from build123d import *

# Parameters (mm, degrees)
F1_DEPTH = 154
F3_D     = 2.7
F3_DEPTH = 12
F3_TIP   = 0.8111618357
F4_W     = 154
F4_H     = 12
F5_DEPTH = 1
F6_W     = 154
F6_H     = 12
F7_DEPTH = 1


with BuildPart() as f1:
    # F0 (on Front) → F1 (new body)
    with BuildSketch(Plane.XZ):
        with BuildLine():
            Line((-10.0352883258, -17.0069661875), (0, -17.0069661875))
            Line((0, -17.0069661875), (10.0352883258, -17.0069661875))
            Line((10.0352883258, -17.0069661875), (7, -12.5069661875))
            Line((7, -12.5069661875), (46.25, -12.5069661875))
            Line((46.25, -12.5069661875), (43.2147116742, -17.0069661875))
            Line((43.2147116742, -17.0069661875), (53.2852883258, -17.0069661875))
            Line((53.2852883258, -17.0069661875), (50.25, -12.5069661875))
            Line((50.25, -12.5069661875), (55.25, -12.5069661875))
            ThreePointArc((55.25, -12.5069661875), (57.3713203436, -11.6282865311), (58.25, -9.5069661875))
            Line((58.25, -9.5069661875), (58.25, 21.9930338125))
            ThreePointArc((58.25, 21.9930338125), (57.3713203436, 24.114354156), (55.25, 24.9930338125))
            Line((55.25, 24.9930338125), (50.8726710718, 24.9930338125))
            Line((50.8726710718, 24.9930338125), (53.5, 20.9930338125))
            Line((53.5, 20.9930338125), (48.25, 20.9930338125))
            Line((48.25, 20.9930338125), (48.25, 4.6930338125))
            Line((48.25, 4.6930338125), (51.35, 4.6930338125))
            Line((51.35, 4.6930338125), (51.35, 1.4930338125))
            Line((51.35, 1.4930338125), (48.25, 1.4930338125))
            Line((48.25, 1.4930338125), (48.25, -3.5069661875))
            ThreePointArc((48.25, -3.5069661875), (47.3713203436, -5.6282865311), (45.25, -6.5069661875))
            Line((45.25, -6.5069661875), (0, -6.5069661875))
            Line((0, -6.5069661875), (-45.25, -6.5069661875))
            ThreePointArc((-45.25, -6.5069661875), (-47.3713203436, -5.6282865311), (-48.25, -3.5069661875))
            Line((-48.25, -3.5069661875), (-48.25, 1.4930338125))
            Line((-48.25, 1.4930338125), (-51.35, 1.4930338125))
            Line((-51.35, 1.4930338125), (-51.35, 4.6930338125))
            Line((-51.35, 4.6930338125), (-48.25, 4.6930338125))
            Line((-48.25, 4.6930338125), (-48.25, 20.9930338125))
            Line((-48.25, 20.9930338125), (-53.5, 20.9930338125))
            Line((-53.5, 20.9930338125), (-50.8726710718, 24.9930338125))
            Line((-50.8726710718, 24.9930338125), (-55.25, 24.9930338125))
            ThreePointArc((-55.25, 24.9930338125), (-57.3713203436, 24.114354156), (-58.25, 21.9930338125))
            Line((-58.25, 21.9930338125), (-58.25, -9.5069661875))
            ThreePointArc((-58.25, -9.5069661875), (-57.3713203436, -11.6282865311), (-55.25, -12.5069661875))
            Line((-55.25, -12.5069661875), (-50.25, -12.5069661875))
            Line((-50.25, -12.5069661875), (-53.2852883258, -17.0069661875))
            Line((-53.2852883258, -17.0069661875), (-43.2147116742, -17.0069661875))
            Line((-43.2147116742, -17.0069661875), (-46.25, -12.5069661875))
            Line((-46.25, -12.5069661875), (-7, -12.5069661875))
            Line((-7, -12.5069661875), (-10.0352883258, -17.0069661875))
        make_face()
        Polygon((-54, -3.1069661875), (-54, -1.4069661875), (-52.4, -1.4069661875), (-52.4, -3.1069661875), (-50.7, -3.1069661875), (-50.7, -4.7069661875), (-52.4, -4.7069661875), (-52.4, -6.4069661875), (-54, -6.4069661875), (-54, -4.7069661875), (-55.7, -4.7069661875), (-55.7, -3.1069661875), align=None, mode=Mode.SUBTRACT)
        Polygon((52.4, -1.4069661875), (54, -1.4069661875), (54, -3.1069661875), (55.7, -3.1069661875), (55.7, -4.7069661875), (54, -4.7069661875), (54, -6.4069661875), (52.4, -6.4069661875), (52.4, -4.7069661875), (50.7, -4.7069661875), (50.7, -3.1069661875), (52.4, -3.1069661875), align=None, mode=Mode.SUBTRACT)
        Polygon((-55.7, 15.5930338125), (-55.7, 17.1930338125), (-54, 17.1930338125), (-54, 18.8930338125), (-52.4, 18.8930338125), (-52.4, 17.1930338125), (-50.7, 17.1930338125), (-50.7, 15.5930338125), (-52.4, 15.5930338125), (-52.4, 13.8930338125), (-54, 13.8930338125), (-54, 15.5930338125), align=None, mode=Mode.SUBTRACT)
        Polygon((54, 18.8930338125), (54, 17.1930338125), (55.7, 17.1930338125), (55.7, 15.5930338125), (54, 15.5930338125), (54, 13.8930338125), (52.4, 13.8930338125), (52.4, 15.5930338125), (50.7, 15.5930338125), (50.7, 17.1930338125), (52.4, 17.1930338125), (52.4, 18.8930338125), align=None, mode=Mode.SUBTRACT)
    extrude(amount=-F1_DEPTH)

    # F3
    with Locations(Plane.XZ):
        with Locations((0, -15.5069661875)):
            Hole(F3_D / 2, depth=F3_DEPTH)
            with Locations((0, 0, -(F3_DEPTH + F3_TIP / 2))):  # 118° drill point
                Cone(0, F3_D / 2, F3_TIP, mode=Mode.SUBTRACT)

    # F4 (on face) → F5 (cut)
    with BuildSketch(Plane.YZ.offset(-48.25)):
        with Locations((77, 3.0930338125)):
            Rectangle(F4_W, F4_H)
    extrude(amount=-F5_DEPTH, mode=Mode.SUBTRACT)

    # F6 (on face) → F7 (cut)
    with BuildSketch(Plane(origin=(48.25, 0, 0), x_dir=(0, -1, 0), z_dir=(-1, 0, 0))):
        with Locations((-77, 3.0930338125)):
            Rectangle(F6_W, F6_H)
    extrude(amount=-F7_DEPTH, mode=Mode.SUBTRACT)


solid = f1.part
Read the model definition and answer for the solid it produces. Units are mm, in the model's axes. A direction names the side the tool comes from. Coordinates: 2 decimals unless noted, no trailing zeros. Write each loop counter-clockwise with the first axis right and the second up, starting at its lowest first coordinate (ties: lowest second). Pieces come first, ordered by that corner, then holes. Notation, with made-up numbers: (18.25, 45) - (37.25, 45) arc R22 cw to (37.25, 70) - close; hole circle Ø5 at (-31.5, -35.5). An arc over 180 degrees is marked (long way). One line per question, with ' | ' between items.
Q1. For faces 4 (the flat face through (0, 154, -7)), 5 (the flat face through (26, 76, -12.507)), 6 (the cylindrical face through (-47.3, 75.9, -5.7)), determine the directions among +Z, -Z, +X, -X, +Y, -Y from which every point of the face is accessible in a straight line to the end or side of a thin tool.
Result set:
face 4: +Z, -Z, +X, -X, +Y | face 5: +Y, -Y | face 6: +Z, +Y, -Y
Q2. Determine the mould class of faces 1 (the cylindrical face through (-57.4, 75.9, -11.6)), 2 (the flat face through (-48.25, 76, 15)), 3 (the flat face through (-51.75, 75.92, -14.73)) for opening direction Z: +Z half, -Z half, draft (parallel to the pull), parting line (faces both ways), or undercut.
Result set:
face 1: -Z half | face 2: draft | face 3: undercut
Q3. Find section A-A, the plane x = -26.5. Write down the section's boundary in (y, z).
Result set:
outline: (0, -12.51) - (154, -12.51) - (154, -6.51) - (0, -6.51) - close
Q4. Each of these flat-tipped pins is pushed along its axis until it touches: P1, Ø5, axis at x = -2.5, y = 37.5, coming from the +Z side; P2, Ø1.3, axis at x = -53.5, y = 51, coming from the -Z side; P3, Ø1.5, axis at x = 27.5, y = 133, coming from the -Z side. Where does it stop, or does it pass through?
Result set:
P1: z = -6.51 | P2: z = -17.01 | P3: z = -12.51
Q5. Consider L1, parallel to X at y = 70.5, z = -3; L2, parallel to X at y = 72, z = -2; L3, parallel to X at y = 15, z = 5.5. Determine where each line is inside the solid, lowest interval first. Write a range as [from, to].
Result set:
L1: [-58.25, -54], [-52.4, -48.25], [48.25, 52.4], [54, 58.25] | L2: [-58.25, -54], [-52.4, -49.25], [49.25, 52.4], [54, 58.25] | L3: [-58.25, -49.25], [49.25, 58.25]
Q6. Find section B-B, the plane y = 31. State how many separate pieces and enclosed holes the cut face has, plus the area to 3 significant figures.
Result set:
separate pieces: 1 | enclosed holes: 4 | area: 1,340 mm^2
